Source: CAD feature listing. Evaluate the final solid. Frame: model axes, mm. A direction names the side the tool comes from. Give positions to 0.01 mm unless a question says otherwise; leave off trailing zeros. Write each loop counter-clockwise with the first axis right and the second up, starting at its lowest first coordinate (ties: lowest second). Pieces come first, ordered by that corner, then holes. Notation, with made-up numbers: (68, -5.5) -> (79, -5.5) arc R32 ccw to (79, 28.5) -> close; hole circle Ø8 at (51.5, -3.5). An arc over 180 degrees is marked (long way). Write item = value, one per line.
from build123d import *

# Parameters (mm, degrees)
SKETCH1_R                       = 1.75
SKETCH1_W                       = 15.9
SKETCH1_H                       = 2.15
MAIN_BODY_DEPTH                 = 2
SKETCH3_W                       = 17.9
SKETCH3_H                       = 2.15
LIGHT_PIPE_SLOT_CUT_DEPTH       = 2
SKETCH4_W                       = 19.9
SKETCH4_H                       = 28
SKETCH4_W_2                     = 17.9
SKETCH4_H_2                     = 2.15
MAIN_BODY_EXTENSION_DEPTH       = 3.3
SKETCH6_W                       = 27.5
SKETCH6_H                       = 0.9
PCB_EDGE_LIP_ONE_SIDE_DEPTH     = 1.5
SKETCH6_3_W                     = 27.5
SKETCH6_3_H                     = 0.9
SKETCH6_3_W_2                   = 28.4
PCB_EDGE_LIP_ANOTHER_SIDE_DEPTH = 1.5
SKETCH8_W                       = 13.9
SKETCH8_H                       = 6.15
SMD_UNDERSIDE_RECESS_DEPTH      = 2
SKETCH9_W                       = 0.95
SKETCH9_H                       = 2.15
LIGHT_PIPE_STOP_DEPTH           = 3.3


with BuildPart() as part:
    # Sketch1 → Main body (new body)
    with BuildSketch(Plane(origin=(0, 0, 0), x_dir=(1, 0, 0), z_dir=(0, 1, 0))):
        Polygon((-2, 15.15), (-2, -4.85), (26.4, -4.85), (26.4, 3.15), (17.9, 3.15), (17.9, 23.15), (-9.6, 23.15), (-9.6, 15.15), align=None)
        with Locations(Location((-5.6, 19.15, 0), (0, 0, 270))):
            Circle(SKETCH1_R, mode=Mode.SUBTRACT)
        with Locations(Location((22.4, -0.85, 0), (0, 0, 270))):
            Circle(SKETCH1_R, mode=Mode.SUBTRACT)
        with Locations((7.95, 1.075)):
            Rectangle(SKETCH1_W, SKETCH1_H, mode=Mode.SUBTRACT)
        with Locations((7.95, 9.075)):
            Rectangle(SKETCH1_W, SKETCH1_H, mode=Mode.SUBTRACT)
        with Locations((7.95, 17.075)):
            Rectangle(SKETCH1_W, SKETCH1_H, mode=Mode.SUBTRACT)
    extrude(amount=MAIN_BODY_DEPTH)

    # Sketch3 → Light pipe slot cut (cut)
    with BuildSketch(Plane(origin=(0, 2, 0), x_dir=(1, 0, 0), z_dir=(0, 1, 0))):
        with Locations((7.95, 17.075)):
            Rectangle(SKETCH3_W, SKETCH3_H)
        with Locations((7.95, 9.075)):
            Rectangle(SKETCH3_W, SKETCH3_H)
        with Locations((7.95, 1.075)):
            Rectangle(SKETCH3_W, SKETCH3_H)
    extrude(amount=-LIGHT_PIPE_SLOT_CUT_DEPTH, mode=Mode.SUBTRACT)

    # Sketch4 → Main body extension (add)
    with BuildSketch(Plane.XZ):
        with Locations((7.95, -9.15)):
            Rectangle(SKETCH4_W, SKETCH4_H)
        with Locations((7.95, -17.075)):
            Rectangle(SKETCH4_W_2, SKETCH4_H_2, mode=Mode.SUBTRACT)
        with Locations((7.95, -9.075)):
            Rectangle(SKETCH4_W_2, SKETCH4_H_2, mode=Mode.SUBTRACT)
        with Locations((7.95, -1.075)):
            Rectangle(SKETCH4_W_2, SKETCH4_H_2, mode=Mode.SUBTRACT)
    extrude(amount=MAIN_BODY_EXTENSION_DEPTH)

    # Sketch6 → PCB edge lip one side (add)
    with BuildSketch(Plane(origin=(0, 2, 0), x_dir=(1, 0, 0), z_dir=(0, 1, 0))):
        with Locations((4.15, 22.7)):
            Rectangle(SKETCH6_W, SKETCH6_H)
    extrude(amount=PCB_EDGE_LIP_ONE_SIDE_DEPTH)

    # Sketch6_3 → PCB edge lip another side (add)
    with BuildSketch(Plane(origin=(0, 2, 0), x_dir=(1, 0, 0), z_dir=(0, 1, 0))):
        with Locations((4.15, 22.7)):
            Rectangle(SKETCH6_3_W, SKETCH6_3_H)
        with Locations((12.2, -4.4)):
            Rectangle(SKETCH6_3_W_2, SKETCH6_3_H)
    extrude(amount=PCB_EDGE_LIP_ANOTHER_SIDE_DEPTH)

    # Sketch8 → SMD underside recess (cut)
    with BuildSketch(Plane(origin=(0, 2, 0), x_dir=(1, 0, 0), z_dir=(0, 1, 0))):
        with Locations((7.95, 17.075)):
            Rectangle(SKETCH8_W, SKETCH8_H)
        with Locations((7.95, 1.075)):
            Rectangle(SKETCH8_W, SKETCH8_H)
        with Locations((7.95, 9.075)):
            Rectangle(SKETCH8_W, SKETCH8_H)
    extrude(amount=-SMD_UNDERSIDE_RECESS_DEPTH, mode=Mode.SUBTRACT)

    # Sketch9 → Light pipe stop (add)
    with BuildSketch(Plane.XZ.offset(3.3)):
        with Locations((-0.525, -1.075)):
            Rectangle(SKETCH9_W, SKETCH9_H)
        with Locations((-0.525, -17.075)):
            Rectangle(SKETCH9_W, SKETCH9_H)
        with Locations((16.425, -1.075)):
            Rectangle(SKETCH9_W, SKETCH9_H)
        with Locations((16.425, -17.075)):
            Rectangle(SKETCH9_W, SKETCH9_H)
        with Locations((-0.525, -9.075)):
            Rectangle(SKETCH9_W, SKETCH9_H)
        with Locations((16.425, -9.075)):
            Rectangle(SKETCH9_W, SKETCH9_H)
    extrude(amount=-LIGHT_PIPE_STOP_DEPTH)


solid = part.part
1) Contact query for flat-ended pins moving along their axis: pin 1 (3 mm diameter, centred on y = 1, z = -17, fed in from +X); pin 2 (1.6 mm diameter, centred on y = 0.5, z = -2.5, fed in from -X); pin 3 (2 mm diameter, centred on x = 11, z = -11.5, fed in from +Y). Output: stop coordinate, or through.
Computed:
pin_1 = 17.9
pin_2 = -2
pin_3 = 2
2) Cut plane C-C (y = -1.5). Return the cut outline in (x, z), then the cut area to 3 significant figures.
Computed:
outline = (-2, -23.15) -> (17.9, -23.15) -> (17.9, 4.85) -> (-2, 4.85) -> close; hole (-0.05, -18.15) -> (15.95, -18.15) -> (15.95, -16) -> (-0.05, -16) -> close; hole (-0.05, -10.15) -> (15.95, -10.15) -> (15.95, -8) -> (-0.05, -8) -> close; hole (-0.05, -2.15) -> (15.95, -2.15) -> (15.95, 0) -> (-0.05, 0) -> close
area = 454 mm²
3) Cut plane B-B (z = 0.85). Return the cut outline in (x, y), then the cut area to 3 significant figures.
Computed:
outline = (-2, -3.3) -> (17.9, -3.3) -> (17.9, 0) -> (20.65, 0) -> (20.65, 2) -> (14.9, 2) -> (14.9, 0) -> (1, 0) -> (1, 2) -> (-2, 2) -> close; (24.15, 0) -> (26.4, 0) -> (26.4, 2) -> (24.15, 2) -> close
area = 87.7 mm²
4) Access query for faces 4 (the flat face through (14.9, 1, -15)), 5 (the flat face through (-8, 0, -19)), 6 (the flat face through (15.95, -2, -1)). Directions: +Z, -Z, +X, -X, +Y, -Y. A direction counts if a zero-diameter tool reaches every point of the face in a straight line with its end or side. Return the directions, or none.
Computed:
face_4 = +Y
face_5 = +Z, -Z, -X, -Y
face_6 = +Y, -Y
5) Cut plane D-D (y = 3). Return the cut outline in (x, z).
Computed:
outline = (-9.6, -23.15) -> (17.9, -23.15) -> (17.9, -22.25) -> (-9.6, -22.25) -> close; (-2, 3.95) -> (26.4, 3.95) -> (26.4, 4.85) -> (-2, 4.85) -> close
6) Draft query along X for faces 1 (the flat face through (9, 0, 4.85)), 2 (the flat face through (8, -1, -8)), 3 (the flat face through (15.95, -2, -9)). Return one class per face: pulls with the +X half, pulls with the -X half, needs draft (parallel to the pull), parting line crosses it, or undercut.
Computed:
face_1 = needs draft
face_2 = undercut
face_3 = undercut
7) Cut plane A-A (x = 8). State how many separate pieces and enclosed holes the cut face has, then the cut area to 3 significant figures.
Computed:
separate_pieces = 4
enclosed_holes = 0
area = 92.9 mm²
8) Material intervals for L1, parallel to X at y = 1.3, z = 0.85; L2, parallel to Z at x = 10, y = -1.5; L3, parallel to X at y = 1.4, z = -19.15, sorted ascending.
Computed:
L1 = -2 to 1, 14.9 to 20.65, 24.15 to 26.4
L2 = -23.15 to -18.15, -16 to -10.15, -8 to -2.15, 0 to 4.85
L3 = -9.6 to -7.35, -3.85 to 1, 14.9 to 17.9
